from build123d import *

# Parameters (mm, degrees)
SKETCH1_W           = 42
SKETCH1_H           = 42
BOSS_EXTRUDE1_DEPTH = 37.25
SKETCH2_R           = 1.5
CUT_EXTRUDE1_DEPTH  = 5
SKETCH3_R           = 11
SKETCH3_R_2         = 9.5
BOSS_EXTRUDE2_DEPTH = 2
BOSS_EXTRUDE3_DEPTH = 23.25
CHAMFER1_SIZE       = 3
SKETCH6_R           = 4.5
CUT_EXTRUDE2_DEPTH  = 3.25
SKETCH7_R           = 2.5
BOSS_EXTRUDE4_DEPTH = 5.75


with BuildPart() as part:
    # Sketch1 → Boss-Extrude1 (new body)
    with BuildSketch(Plane(origin=(0, 0, 0), x_dir=(1, 0, 0), z_dir=(0, 1, 0))):
        Rectangle(SKETCH1_W, SKETCH1_H)
    extrude(amount=BOSS_EXTRUDE1_DEPTH)

    # Sketch2 → Cut-Extrude1 (cut)
    with BuildSketch(Plane(origin=(0, 37.25, 0), x_dir=(1, 0, 0), z_dir=(0, 1, 0))):
        with Locations((15.5, 15.5)):
            Circle(SKETCH2_R)
        with Locations((15.5, -15.5)):
            Circle(SKETCH2_R)
        with Locations((-15.5, -15.5)):
            Circle(SKETCH2_R)
        with Locations((-15.5, 15.5)):
            Circle(SKETCH2_R)
    extrude(amount=-CUT_EXTRUDE1_DEPTH, mode=Mode.SUBTRACT)

    # Sketch3 → Boss-Extrude2 (add)
    with BuildSketch(Plane(origin=(0, 37.25, 0), x_dir=(1, 0, 0), z_dir=(0, 1, 0))):
        Circle(SKETCH3_R)
        Circle(SKETCH3_R_2, mode=Mode.SUBTRACT)
    extrude(amount=BOSS_EXTRUDE2_DEPTH)

    # Chamfer1
    chamfer1_edges = [part.edges().sort_by_distance(p)[0] for p in [
        (21, 18.625, 21),
        (-21, 18.625, 21),
        (-21, 18.625, -21),
        (21, 18.625, -21),
    ]]
    chamfer(chamfer1_edges, length=CHAMFER1_SIZE)

    # Sketch6 → Cut-Extrude2 (cut)
    with BuildSketch(Plane.XZ):
        Circle(SKETCH6_R)
    extrude(amount=-CUT_EXTRUDE2_DEPTH, mode=Mode.SUBTRACT)



with BuildPart() as body_2:
    # Sketch4 → Boss-Extrude3 (new body)
    with BuildSketch(Plane(origin=(0, 60.5, 0), x_dir=(1, 0, 0), z_dir=(0, 1, 0))):
        with BuildLine():
            Line((-1.275735082, -2.15), (1.275735082, -2.15))
            ThreePointArc((1.275735082, -2.15), (0, 2.5), (-1.275735082, -2.15))
        make_face()
    extrude(amount=-BOSS_EXTRUDE3_DEPTH)


with BuildPart() as part_1:
    add(part.part)

    add(body_2.part)  # Boss-Extrude4 merges body 2
    # Sketch7 → Boss-Extrude4 (add)
    with BuildSketch(Plane(origin=(0, 37.25, 0), x_dir=(1, 0, 0), z_dir=(0, 1, 0))):
        Circle(SKETCH7_R)
    extrude(amount=BOSS_EXTRUDE4_DEPTH)


solid = part_1.part
For this review, take the finished solid that the model builds, in its own axes (mm). A direction names the side the tool comes from. Coordinates: 2 decimals unless noted, no trailing zeros. Loops run counter-clockwise (first coordinate to the right, second up) from the corner with the lowest first, then second, coordinate; pieces in that order, holes last. Notation, with made-up numbers: (44.5, 51.5) - (79.5, 51.5) arc R10 ccw to (79.5, 60.5) - close; hole circle Ø9 at (34.25, 31.5). An arc over 180 degrees is marked (long way). Return JSON: item names as keys, results as strings.
Item 1: Take a section at B-B (z = 0). Give the boundary of the cut face in (x, y), then the cut area to 3 significant figures.
Determined:
{"outline": "(-21, 0) - (-4.5, 0) - (-4.5, 3.25) - (4.5, 3.25) - (4.5, 0) - (21, 0) - (21, 37.25) - (11, 37.25) - (11, 39.25) - (9.5, 39.25) - (9.5, 37.25) - (2.5, 37.25) - (2.5, 60.5) - (-2.5, 60.5) - (-2.5, 37.25) - (-9.5, 37.25) - (-9.5, 39.25) - (-11, 39.25) - (-11, 37.25) - (-21, 37.25) - close", "area": "1,660 mm2"}
Item 2: Take a section at C-C (y = 38). Give the boundary of the cut face in (x, z), then the cut area to 3 significant figures.
Determined:
{"outline": "circle Ø22 at (0, 0); circle Ø5 at (0, 0); hole circle Ø19 at (0, 0)", "area": "116 mm2"}
Item 3: Mouldability with a two-part tool opening along X and no side actions: class faces 6 (the flat face through (-21, 18, 0)), 7 (the flat face through (21, 18, 0)), 8 (the cylindrical face through (4.38, 38.24, 8.43)), 9 (the flat face through (0, 18, -21)) as pulls with the +X half, pulls with the -X half, needs draft (parallel to the pull), parting line crosses it, or undercut.
Determined:
{"face 6": "pulls with the -X half", "face 7": "pulls with the +X half", "face 8": "undercut", "face 9": "needs draft"}
Item 4: Take a section at A-A (x = 0). Give the boundary of the cut face in (y, z), then the cut area to 3 significant figures.
Determined:
{"outline": "(0, -21) - (37.25, -21) - (37.25, -11) - (39.25, -11) - (39.25, -9.5) - (37.25, -9.5) - (37.25, -2.5) - (60.5, -2.5) - (60.5, 2.15) - (43, 2.15) - (43, 2.5) - (37.25, 2.5) - (37.25, 9.5) - (39.25, 9.5) - (39.25, 11) - (37.25, 11) - (37.25, 21) - (0, 21) - (0, 4.5) - (3.25, 4.5) - (3.25, -4.5) - (0, -4.5) - close", "area": "1,650 mm2"}
Item 5: For line 1 (X direction, y = 35.25, z = -15.5); line 2 (Z direction, x = 0, y = 38.6), list the stretches that pass through material, from the lowest coordinate up.
Determined:
{"line 1": "x = -21 to -17, -14 to 14, 17 to 21", "line 2": "z = -11 to -9.5, -2.5 to 2.5, 9.5 to 11"}
Item 6: Insertion check: pin 1 (11.5 mm diameter, centred on x = 0, z = 0, fed in from -Y); pin 2 (3 mm diameter, centred on x = -0.5, y = 53, fed in from +Z); pin 3 (3.5 mm diameter, centred on x = -15.5, z = 16, fed in from +Y); pin 4 (2.5 mm diameter, centred on x = -2, z = -0.5, fed in from -Y). Each pin has a flat end and moves straight along its axis. Give the tip position at first contact, or say it passes through.
Determined:
{"pin 1": "stops at y = 0", "pin 2": "stops at z = 2.15", "pin 3": "stops at y = 37.25", "pin 4": "stops at y = 3.25"}
Item 7: For faces 1 (the flat face through (0, 3.25, 0)), 2 (the flat face through (0, 18, 21)), 3 (the flat face through (0, 0, -5)), 4 (the flat face through (2, 37.25, 2)), 5 (the flat face through (0, 52, 2.15)), list the 3-axis set-ups (+Z, -Z, +X, -X, +Y, -Y) from which the entire face can be reached by the end or side of a thin tool; tool diameter is ignored.
Determined:
{"face 1": "-Y", "face 2": "+Z, +X, -X, +Y, -Y", "face 3": "+Z, -Z, +X, -X, -Y", "face 4": "+Y", "face 5": "+Z, +X, -X, +Y"}
Item 8: Take a section at D-D (x = 15.5). Give the boundary of the cut face in (y, z), then the cut area to 3 significant figures.
Determined:
{"outline": "(0, -21) - (37.25, -21) - (37.25, -17) - (32.25, -17) - (32.25, -14) - (37.25, -14) - (37.25, 14) - (32.25, 14) - (32.25, 17) - (37.25, 17) - (37.25, 21) - (0, 21) - close", "area": "1,530 mm2"}
